from build123d import *

# Parameters (mm, degrees)
F1_DEPTH = 482.6
F2_R     = 12.2642048969
F5_D     = 5.08


with BuildPart() as f1:
    # F0 (on Front) → F1 (new body)
    with BuildSketch(Plane.XZ):
        Polygon((25.4, 12.7), (-25.4, 12.7), (-10.7353031626, -12.7), (10.7353031626, -12.7), align=None)
    extrude(amount=-F1_DEPTH)

    # F2
    f2_edges = [f1.edges().sort_by_distance(p)[0] for p in [
        (0, 482.6, 12.7),
        (18.067652, 482.6, 0),
        (0, 482.6, -12.7),
        (-18.067652, 482.6, 0),
    ]]
    fillet(f2_edges, radius=F2_R)

    # F5 (through all)
    with Locations(Plane.XY.offset(12.7)):
        with Locations((0, 330.2), (0, 50.8)):
            Hole(F5_D / 2)


solid = f1.part
Work out the finished part from the listing and answer in its coordinate system (mm). Round coordinates to 2 decimals unless told otherwise and drop trailing zeros. Loops run counter-clockwise (first coordinate to the right, second up) from the corner with the lowest first, then second, coordinate; pieces in that order, holes last. Notation, with made-up numbers: (48, 71.25) - (101, 71.25) arc R27 cw to (101, 90.25) - close; hole circle Ø10 at (29.25, -23.5). An arc over 180 degrees is marked (long way). One line per item, written item: value.
Q1. Each of these flat-tipped pins is pushed along its axis until it touches: pin 1 Ø10 at (y, z) = (177.5, -8.5) entering from -X; pin 2 Ø12 at (y, z) = (105, 1.5) entering from -X; pin 3 Ø4.5 at (x, y) = (0, 330.2) entering from -Z (3 decimals); pin 4 Ø2 at (x, y) = (-19, 325.5) entering from -Z. Where does it stop, or does it pass through?
Check values:
pin 1: x = -16.05
pin 2: x = -22.4
pin 3: through
pin 4: z = -0.12
Q2. Find section A-A on y = 281.5. Give the vertices of the cut face in (x, z), and give its area (3 significant figures).
Check values:
outline: (-25.4, 12.7) - (-10.74, -12.7) - (10.74, -12.7) - (25.4, 12.7) - close
area: 918 mm2
Q3. Straight lines are drawn through the part: probe 1 along Y at (x, z) = (0, -0.5); probe 2 along Y at (x, z) = (0, 3.75); probe 3 along Z at (x, y) = (20.5, 408.5). For each, find the intervals that lie inside material, in ascending order.
Check values:
probe 1: 0 to 48.26, 53.34 to 327.66, 332.74 to 482.6
probe 2: 0 to 48.26, 53.34 to 327.66, 332.74 to 482.14
probe 3: 4.21 to 12.7
Q4. Find section B-B on z = -4.75. State how many separate pieces and enclosed holes the cut face has, and give its area (3 significant figures).
Check values:
separate pieces: 1
enclosed holes: 2
area: 14,700 mm2
